For this review, take the finished solid that the model builds, in its own axes (mm). A direction names the side the tool comes from. Give positions to 0.01 mm unless a question says otherwise; leave off trailing zeros. Loops run counter-clockwise (first coordinate to the right, second up) from the corner with the lowest first, then second, coordinate; pieces in that order, holes last. Notation, with made-up numbers: (-31, 12) -> (-5, 12) arc R12 ccw to (-5, 29) -> close; hole circle Ø3 at (45, 68). An arc over 180 degrees is marked (long way). One line per question, with ' | ' between items. Start each with the question number.
(1) Consider section C-C (y = -30). Write out the cut boundary in (x, z).
(2) Consider section B-B (y = 0). Write out the cut boundary in (x, z), and give its area (3 significant figures).
(3) Draft analysis for pull direction X (two halves, no side actions). For faces 1 (the cylindrical face through (-31.84, 31.69, 2.96)), 2 (the cylindrical face through (28.16, 31.69, 2.96)), 3 (the flat face through (40.5, 10, 3)), 4 (the flat face through (-57.81, 30.5, 2.96)), state which applies: +X half, -X half, draft (parallel to the pull), parting line (faces both ways), or undercut.
(4) Tool access review of faces 5 (the flat face through (29, -10, 3)), 6 (the cylindrical face through (-27.91, -40.29, 2.96)): name each direction out of +Z, -Z, +X, -X, +Y, -Y from which nothing blocks a thin tool from reaching the whole face with its end or side.
(5) Consider section D-D (x = -65). Write out the cut boundary in (y, z).
(6) Consider section A-A (z = 4.9). Give the number of separate pieces and of enclosed holes in the cut face, and give its area (3 significant figures).
(7) Wall thickness on probe 1 along Y at (x, z) = (30, 2.25); probe 2 along Y at (x, z) = (-30, 2.6); probe 3 along Y at (x, z) = (-80, 4): over which ranges is each line inside the solid? List them lowest first.
(8) Insertion check: P1, Ø3, axis at x = -80.35, y = -15.35, coming from the -Z side; P2, Ø2, axis at x = -22.5, z = 3, coming from the -Y side; P3, Ø3, axis at x = 26, z = 4, coming from the -Y side. Each pin has a flat end and moves straight along its axis. Give the tip position at first contact, or say it passes through.
from build123d import *

# Parameters (mm, degrees)
ESBO_O1_R                = 2.5
ESBO_O1_R_2              = 1.75
ESBO_O1_R_3              = 11
ESBO_O1_R_4              = 2
RESSALTO_EXTRUS_O1_DEPTH = 6


with BuildPart() as part:
    # Esboço1 → Ressalto-extrusão1 (new body)
    with BuildSketch(Plane.XY):
        with BuildLine():
            Line((-22.575378798, -37.424621202), (-3.937554159, -18.786796564))
            ThreePointArc((-3.937554159, -18.786796564), (5.795146305, -12.283614025), (17.275649276, -10))
            Line((17.275649276, -10), (40.5, -10))
            Line((40.5, -10), (40.5, 30))
            ThreePointArc((40.5, 30), (37.424621202, 37.424621202), (30, 40.5))
            Line((30, 40.5), (-30, 40.5))
            ThreePointArc((-30, 40.5), (-31.926738888, 40.321709028), (-33.788045366, 39.792890906))
            Line((-33.788045366, 39.792890906), (-82.513696647, 20.945036955))
            ThreePointArc((-82.513696647, 20.945036955), (-85.298219626, 18.741179474), (-86.349099295, 15.349099295))
            Line((-86.349099295, 15.349099295), (-86.349099295, -15.349099295))
            ThreePointArc((-86.349099295, -15.349099295), (-85.298219626, -18.741179474), (-82.513696647, -20.945036955))
            Line((-82.513696647, -20.945036955), (-33.788045366, -39.792890906))
            ThreePointArc((-33.788045366, -39.792890906), (-27.830127584, -40.273346762), (-22.575378798, -37.424621202))
        make_face()
        with Locations((-30, 30)):
            Circle(ESBO_O1_R, mode=Mode.SUBTRACT)
        with Locations((-30, -30)):
            Circle(ESBO_O1_R, mode=Mode.SUBTRACT)
        with Locations((30, 30)):
            Circle(ESBO_O1_R, mode=Mode.SUBTRACT)
        with Locations((-80.349099295, 15.349099295)):
            Circle(ESBO_O1_R_2, mode=Mode.SUBTRACT)
        with Locations((-49.650900705, 15.349099295)):
            Circle(ESBO_O1_R_2, mode=Mode.SUBTRACT)
        with Locations((-49.650900705, -15.349099295)):
            Circle(ESBO_O1_R_2, mode=Mode.SUBTRACT)
        with Locations((-80.349099295, -15.349099295)):
            Circle(ESBO_O1_R_2, mode=Mode.SUBTRACT)
        with Locations((-65, 0)):
            Circle(ESBO_O1_R_3, mode=Mode.SUBTRACT)
        with Locations((-30, 0)):
            Circle(ESBO_O1_R_4, mode=Mode.SUBTRACT)
        with Locations((30, 0)):
            Circle(ESBO_O1_R_4, mode=Mode.SUBTRACT)
    extrude(amount=RESSALTO_EXTRUS_O1_DEPTH)


solid = part.part
A:
1) outline: (-59.1, 0) -> (-32.5, 0) -> (-32.5, 6) -> (-59.1, 6) -> close; (-27.5, 0) -> (-15.15, 0) -> (-15.15, 6) -> (-27.5, 6) -> close
2) outline: (-86.35, 0) -> (-76, 0) -> (-76, 6) -> (-86.35, 6) -> close; (-54, 0) -> (-32, 0) -> (-32, 6) -> (-54, 6) -> close; (-28, 0) -> (28, 0) -> (28, 6) -> (-28, 6) -> close; (32, 0) -> (40.5, 0) -> (40.5, 6) -> (32, 6) -> close | area: 581 mm^2
3) face 1: undercut | face 2: undercut | face 3: +X half | face 4: -X half
4) face 5: +Z, -Z, +X, -Y | face 6: +Z, -Z, -Y
5) outline: (-27.72, 0) -> (-11, 0) -> (-11, 6) -> (-27.72, 6) -> close; (11, 0) -> (27.72, 0) -> (27.72, 6) -> (11, 6) -> close
6) separate pieces: 1 | enclosed holes: 10 | area: 7,060 mm^2
7) probe 1: y = -10 to -2, 2 to 27.5, 32.5 to 40.5 | probe 2: y = -40.5 to -32.5, -27.5 to -2, 2 to 27.5, 32.5 to 40.5 | probe 3: y = -21.92 to -17.06, -13.63 to 13.63, 17.06 to 21.92
8) P1: passes through | P2: stops at y = -38.25 | P3: stops at y = -10
